from build123d import *

# Parameters (mm, degrees)
SKETCH1_R           = 4.25
BOSS_EXTRUDE4_DEPTH = 3.2
SKETCH3_W           = 1
SKETCH3_H           = 4
SKETCH3_W_2         = 4
SKETCH3_H_2         = 1
CUT_EXTRUDE1_DEPTH  = 0.5
SKETCH4_R           = 2.5
BOSS_EXTRUDE7_DEPTH = 10


with BuildPart() as part:
    # Sketch1 → Boss-Extrude4 (new body)
    with BuildSketch(Plane.XY):
        Circle(SKETCH1_R)
    extrude(amount=BOSS_EXTRUDE4_DEPTH)

    # Sketch2 → Cut-Revolve1 (revolve, cut)
    with BuildSketch(Plane(origin=(0, 0, 0), x_dir=(1, 0, 0), z_dir=(0, 1, 0))):
        with BuildLine():
            Line((-4.25, -1.6), (-4.25, 0))
            Line((-4.25, 0), (-2.65, 0))
            ThreePointArc((-2.65, 0), (-3.78137085, -0.46862915), (-4.25, -1.6))
        make_face()
    revolve(axis=Axis((0, 0, 0), (0, 0, 1)), mode=Mode.SUBTRACT)

    # Sketch3 → Cut-Extrude1 (cut)
    with BuildSketch(Plane(origin=(0, 0, 0), x_dir=(-1, 0, 0), z_dir=(0, 0, -1))):
        Rectangle(SKETCH3_W, SKETCH3_H)
        Rectangle(SKETCH3_W_2, SKETCH3_H_2)
    extrude(amount=-CUT_EXTRUDE1_DEPTH, mode=Mode.SUBTRACT)

    # Sketch4 → Boss-Extrude7 (add)
    with BuildSketch(Plane.XY.offset(3.2)):
        Circle(SKETCH4_R)
    extrude(amount=BOSS_EXTRUDE7_DEPTH)


solid = part.part
Model file for the job. Use its own axes, mm. A direction names the side the tool comes from. Give positions to 0.01 mm unless a question says otherwise; leave off trailing zeros. Loops run counter-clockwise (first coordinate to the right, second up) from the corner with the lowest first, then second, coordinate; pieces in that order, holes last.
1) Tool access for faces 4 (the cylindrical face through (2.285, 3.584, 2.389)), 5 (the flat face through (2, -2, 3.2)): list every direction of +Z, -Z, +X, -X, +Y, -Y with a clear straight run to the whole face (end or side of a thin tool).
2) Saw through at A-A (y = 0). Write the cut outline in (x, z).
3) Flat gauge pin, fed straight in: pin 1 Ø0.6 at (y, z) = (-1.5, 0.5) entering from -X. Where does the tip first touch, or does it go through?
4) Saw through at C-C (z = 2.5). Write the cut outline in (x, y), plus the area to 3 significant figures.
5) Saw through at D-D (z = 6.5). Write the cut outline in (x, y), plus the area to 3 significant figures.
6) Wall check: line 1 (Y direction, x = 0, z = 7.25); line 2 (Z direction, x = 0.5, y = 0); line 3 (X direction, y = -3.5, z = 1.25). Give the ranges that are in metal, low to high.
7) Pull direction X, two halves, no side cores. Call faces 1 (the flat face through (1, -1, 0)), 2 (the cylindrical face through (-0.54, -2.44, 8.13)), 3 (the flat face through (0, 0, 0.5)): +X half, -X half, draft (parallel to the pull), parting line (faces both ways), or undercut.
Answer block:
1. face 4: +Z, -Z
1. face 5: +Z
2. outline: (-4.25, 1.6) arc R1.6 ccw to (-2.65, 0) - (-2, 0) - (-2, 0.5) - (2, 0.5) - (2, 0) - (2.65, 0) arc R1.6 ccw to (4.25, 1.6) - (4.25, 3.2) - (2.5, 3.2) - (2.5, 13.2) - (-2.5, 13.2) - (-2.5, 3.2) - (-4.25, 3.2) - close
3. pin 1: stops at x = -3.78
4. outline: circle Ø8.5 at (0, 0)
4. area: 56.7 mm2
5. outline: circle Ø5 at (0, 0)
5. area: 19.6 mm2
6. line 1: y = -2.5 to 2.5
6. line 2: z = 0.5 to 13.2
6. line 3: x = -2.34 to 2.34
7. face 1: draft
7. face 2: parting line
7. face 3: undercut
